```python
from build123d import *

# Parameters (mm, degrees)
F0_W          = 120
F0_H          = 50
F1_DEPTH      = 25
F1_DEPTH_BACK = 25
F3_R          = 12.7


with BuildPart() as f1:
    # F0 (on Front) → F1 (new body, two sides)
    with BuildSketch(Plane.XZ) as f1_sk:
        with Locations((42.842679834, -25)):
            Rectangle(F0_W, F0_H)
    extrude(amount=F1_DEPTH)
    extrude(f1_sk.sketch, amount=-F1_DEPTH_BACK)

    # F4: sweep along a path in F2
    with BuildLine(Plane.XZ) as f4_path:
        Line((0, 0), (0, 150))
        Line((0, 150), (-750, 150))
        Line((-750, 150), (-750, 920))
        Line((-750, 920), (-950, 920))
    # F3 (on Top) → F4 (sweep)
    with BuildSketch(Plane.XY):
        Circle(F3_R)
    sweep(path=f4_path.line, transition=Transition.RIGHT)


solid = f1.part
```
Verification items for the finished model (mm, model axes). A direction names the side the tool comes from. Coordinates: 2 decimals unless noted, no trailing zeros. Write each loop counter-clockwise with the first axis right and the second up, starting at its lowest first coordinate (ties: lowest second). Pieces come first, ordered by that corner, then holes. Notation, with made-up numbers: (30, 39.25) - (61, 39.25) arc R19 ccw to (61, 70.25) - close; hole circle Ø9 at (29.25, -24.5). An arc over 180 degrees is marked (long way). One line per question, with ' | ' between items. Start each with the question number.
1. Section check A-A (y = 0). Enter the section's corners in (x, z), plus the area to 3 significant figures.
2. Section check D-D (x = -750). Enter the section's corners in (y, z).
3. Section check B-B (x = 0). Enter the section's corners in (y, z).
4. Gauge pin test, flat ends, axial feed: P1, Ø8, axis at y = 3.5, z = 635, coming from the +X side; P2, Ø2, axis at x = -795.5, y = 1.5, coming from the +Z side; P3, Ø6, axis at y = -11.5, z = 83.5, coming from the +X side. Record the tip position at first contact, or that the pin passes through.
5. Material ranges on line 1 along Z through (x, y) = (-490, 0); line 2 along X through (y, z) = (10, -9.5); line 3 along Z through (x, y) = (-688, -11), recorded low to high.
6. Section check C-C (z = 768). Enter the section's corners in (x, y).
7. Access from +Z, -Z, +X, -X, +Y, -Y to the whole of each face (thin tool, end or side, straight path). Record for faces 4 (the cylindrical face through (-845.139, -4.864, 931.732)), 5 (the flat face through (-17.157, 0, -25)), 6 (the flat face through (42, -25, -25)), 7 (the cylindrical face through (-762.688, 0.558, 540.568)), 8 (the flat face through (42, 25, -25)).
8. Draft check along Z on faces 1 (the flat face through (102.843, 0, -25)), 2 (the flat face through (42, 0, -50)), 3 (the cylindrical face through (12.114, 3.815, 82.489)). Enter one of: released by +Z, released by -Z, zero draft, split by the parting line, or undercut.
Computed values:
1) outline: (-950, 907.3) - (-762.7, 907.3) - (-762.7, 137.3) - (-12.7, 137.3) - (-12.7, 0) - (-17.16, 0) - (-17.16, -50) - (102.84, -50) - (102.84, 0) - (12.7, 0) - (12.7, 162.7) - (-737.3, 162.7) - (-737.3, 932.7) - (-950, 932.7) - close | area: 53,500 mm²
2) outline: (-12.7, 150) arc R12.7 ccw to (12.7, 150) - (12.7, 920) arc R12.7 ccw to (-12.7, 920) - close
3) outline: (-25, -50) - (25, -50) - (25, 0) - (12.7, 0) - (12.7, 150) arc R12.7 ccw to (-12.7, 150) - (-12.7, 0) - (-25, 0) - close
4) P1: x = -737.3 | P2: z = 932.69 | P3: x = 9.44
5) line 1: 137.3 to 162.7 | line 2: -17.16 to 102.84 | line 3: 143.65 to 156.35
6) outline: circle Ø25.4 at (-750, 0)
7) face 4: -X | face 5: -Z, -X, +Y, -Y | face 6: +Z, -Z, +X, -X, -Y | face 7: none | face 8: +Z, -Z, +X, -X, +Y
8) face 1: zero draft | face 2: released by -Z | face 3: undercut
